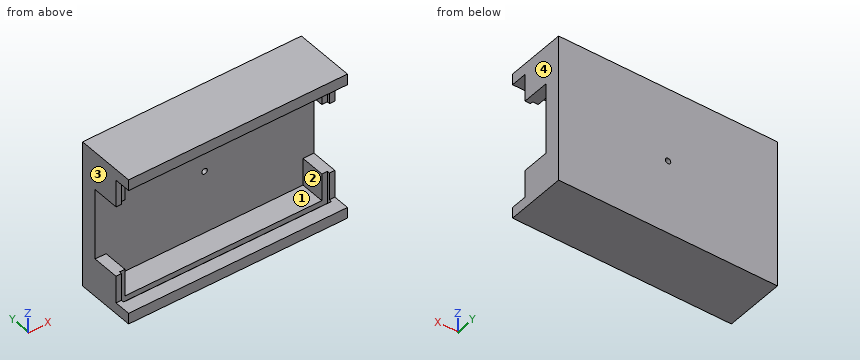
```python
from build123d import *

# Parameters (mm, degrees)
SKETCH3_W           = 40
SKETCH3_H           = 40
SKETCH3_R           = 5
SKETCH3_R_2         = 0.5
BOSS_EXTRUDE2_DEPTH = 3
BOSS_EXTRUDE3_DEPTH = 8
SKETCH6_W           = 2
SKETCH6_H           = 5
BOSS_EXTRUDE5_DEPTH = 5
SKETCH7_W           = 40
SKETCH7_H           = 6.5
CUT_EXTRUDE1_DEPTH  = 3
SKETCH8_W           = 40
SKETCH8_H           = 6.5
CUT_EXTRUDE2_DEPTH  = 3
CUT_EXTRUDE3_START  = -1
SKETCH5_W           = 5
SKETCH5_H           = 0.5
CUT_EXTRUDE3_DEPTH  = 6


with BuildPart() as part:
    # Sketch3 → Boss-Extrude2 (new body)
    with BuildSketch(Plane(origin=(0, 0, 0), x_dir=(1, 0, 0), z_dir=(0, 1, 0))):
        Rectangle(SKETCH3_W, SKETCH3_H)
        Circle(SKETCH3_R, mode=Mode.SUBTRACT)
        Circle(SKETCH3_R)
        Circle(SKETCH3_R_2, mode=Mode.SUBTRACT)
    extrude(amount=-BOSS_EXTRUDE2_DEPTH)

    # Sketch4 → Boss-Extrude3 (add)
    with BuildSketch(Plane.XZ.offset(3)):
        Polygon((20, -11.5), (0, -11.5), (-20, -11.5), (-20, -13.5), (20, -13.5), align=None)
        Polygon((-20, 11.5), (0, 11.5), (20, 11.5), (20, 13.5), (-20, 13.5), align=None)
    extrude(amount=BOSS_EXTRUDE3_DEPTH)

    # Sketch6 → Boss-Extrude5 (add)
    with BuildSketch(Plane.XZ.offset(3)):
        with Locations((19, 9)):
            Rectangle(SKETCH6_W, SKETCH6_H)
        with Locations((19, -9)):
            Rectangle(SKETCH6_W, SKETCH6_H)
        with Locations((-19, -9)):
            Rectangle(SKETCH6_W, SKETCH6_H)
        with Locations((-19, 9)):
            Rectangle(SKETCH6_W, SKETCH6_H)
    extrude(amount=BOSS_EXTRUDE5_DEPTH)

    # Sketch7 → Cut-Extrude1 (cut)
    with BuildSketch(Plane(origin=(0, -3, 0), x_dir=(-1, 0, 0), z_dir=(0, -1, 0))):
        with Locations((0, -16.75)):
            Rectangle(SKETCH7_W, SKETCH7_H)
    extrude(amount=-CUT_EXTRUDE1_DEPTH, mode=Mode.SUBTRACT)

    # Sketch8 → Cut-Extrude2 (cut)
    with BuildSketch(Plane.XZ.offset(3)):
        with Locations((0, -16.75)):
            Rectangle(SKETCH8_W, SKETCH8_H)
    extrude(amount=-CUT_EXTRUDE2_DEPTH, mode=Mode.SUBTRACT)

    # Sketch5 → Cut-Extrude3 (cut)
    with BuildSketch(Plane.XY.offset(-11.5).offset(CUT_EXTRUDE3_START)):
        Polygon((19, -7.5), (0, -7.5), (0, -8), (5, -8), (5, -8.5), (19, -8.5), align=None)
        Polygon((0, -8), (0, -7.5), (-19, -7.5), (-19, -8.5), (-5, -8.5), (-5, -8), align=None)
        with Locations((-2.5, -8.25)):
            Rectangle(SKETCH5_W, SKETCH5_H)
        with Locations((2.5, -8.25)):
            Rectangle(SKETCH5_W, SKETCH5_H)
    cut_extrude3 = extrude(amount=CUT_EXTRUDE3_DEPTH, mode=Mode.SUBTRACT)

    # Mirror2: Cut-Extrude3 across plane
    add(cut_extrude3.mirror(Plane.XY), mode=Mode.SUBTRACT)


solid = part.part
```
For this review, take the finished solid that the model builds, in its own axes (mm). Face numbers are marked on the shaded views. Round coordinates to 2 decimals unless told otherwise and drop trailing zeros. Write each loop counter-clockwise with the first axis right and the second up, starting at its lowest first coordinate (ties: lowest second). Pieces come first, ordered by that corner, then holes. Notation, with made-up numbers: (75.5, -27.5) - (101.5, -27.5) arc R28 cw to (101.5, -2.5) - close; hole circle Ø8 at (35.25, 2.25). An arc over 180 degrees is marked (long way). Answer as a JSON object with one key per item and string values.
1. To check wall thickness, follow line 1 along Z through (x, y) = (-9, -7.75); line 2 along Z through (x, y) = (14.5, -5); line 3 along X through (y, z) = (-0.85, 0). State the ranges of each line that lie inside material, in increasing order.
Response values:
{"line 1": "z = -13.5 to -12.5, 12.5 to 13.5", "line 2": "z = -13.5 to -11.5, 11.5 to 13.5", "line 3": "x = -20 to -0.5, 0.5 to 20"}
2. We need section A-A on x = 0. Give the boundary of the cut face in (y, z), then the cut area to 3 significant figures.
Response values:
{"outline": "(-11, -13.5) - (0, -13.5) - (0, -0.5) - (-3, -0.5) - (-3, -11.5) - (-7.5, -11.5) - (-7.5, -12.5) - (-8.5, -12.5) - (-8.5, -11.5) - (-11, -11.5) - close; (-11, 11.5) - (-8.5, 11.5) - (-8.5, 12.5) - (-7.5, 12.5) - (-7.5, 11.5) - (-3, 11.5) - (-3, 0.5) - (0, 0.5) - (0, 13.5) - (-11, 13.5) - close", "area": "108 mm2"}
3. We need section C-C on y = -5.5. Give the boundary of the cut face in (x, z), then the cut area to 3 significant figures.
Response values:
{"outline": "(-20, -13.5) - (20, -13.5) - (20, -6.5) - (18, -6.5) - (18, -11.5) - (-18, -11.5) - (-18, -6.5) - (-20, -6.5) - close; (-20, 6.5) - (-18, 6.5) - (-18, 11.5) - (18, 11.5) - (18, 6.5) - (20, 6.5) - (20, 13.5) - (-20, 13.5) - close", "area": "200 mm2"}
4. We need section D-D on x = 5.5. Give the boundary of the cut face in (y, z).
Response values:
{"outline": "(-11, -13.5) - (0, -13.5) - (0, 13.5) - (-11, 13.5) - (-11, 11.5) - (-8.5, 11.5) - (-8.5, 12.5) - (-7.5, 12.5) - (-7.5, 11.5) - (-3, 11.5) - (-3, -11.5) - (-7.5, -11.5) - (-7.5, -12.5) - (-8.5, -12.5) - (-8.5, -11.5) - (-11, -11.5) - close"}
5. We need section B-B on z = 0. Give the boundary of the cut face in (x, y).
Response values:
{"outline": "(-20, -3) - (-0.5, -3) - (-0.5, 0) - (-20, 0) - close; (0.5, -3) - (20, -3) - (20, 0) - (0.5, 0) - close"}
6. For pin 1 Ø8 at (x, z) = (15.5, 10) entering from -Y; pin 2 Ø5 at (y, z) = (-9.5, 2.5) entering from +X, all flat-tipped, find the tip position at first contact; note any pin that passes through.
Response values:
{"pin 1": "stops at y = -11", "pin 2": "passes through"}
7. Draft analysis for pull direction X (two halves, no side actions). For the marked faces 1, 2, 3 and 4, state which applies: +X half, -X half, draft (parallel to the pull), parting line (faces both ways), or undercut.
Response values:
{"face 1": "undercut", "face 2": "undercut", "face 3": "-X half", "face 4": "+X half"}
